Here's the drawing with two shaded views (mm, measured from the low corner). I have some questions. A direction names the side the tool comes from. Coordinates: 2 decimals unless noted, no trailing zeros. Order: outer loops, then holes, each group sorted by start corner. A loop starts at its lowest first (then second) coordinate and runs counter-clockwise, first axis right, second up. Notation, with made-up numbers: M -1.5,2 L 44.5,2 A27 cw 44.5,35 Z; hole C 21,-15.75 d11. An arc over 180 degrees is marked long. Put each result on its own line as item: value. Start each with the question number.
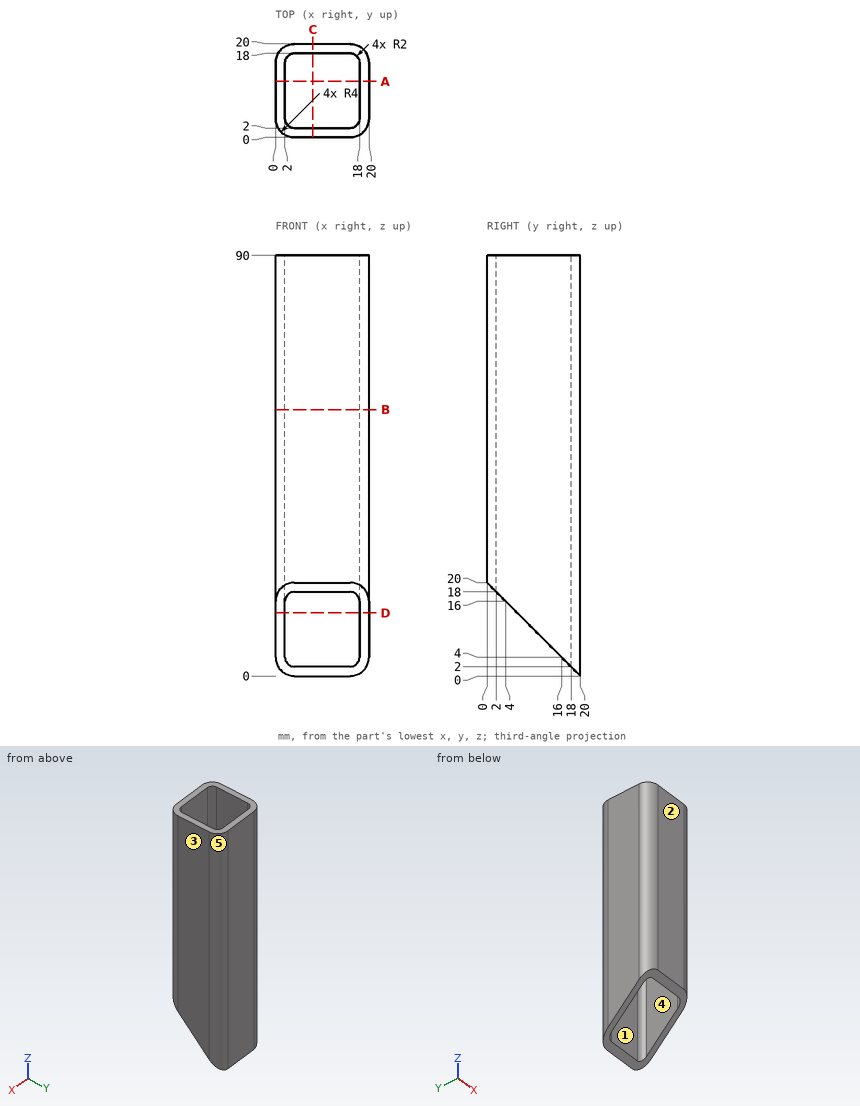
Item 1: If we section it at A-A on y = 12: Write out the boundary of the cut face in (x, z), then the cut area to 3 significant figures.
Item 2: If we section it at D-D on z = 13.5: Write out the boundary of the cut face in (x, y), then the cut area to 3 significant figures.
Item 3: If we mould it in two halves opening along Y, with no side actions, what happens to the marked faces 3, 4 and 5? For each: released by +Y, released by -Y, zero draft, split by the parting line, or undercut.
Item 4: If we section it at B-B on z = 57: Write out the boundary of the cut face in (x, y), then the cut area to 3 significant figures.
Item 5: I need wall thicknesses on probe 1 along Y at (x, z) = (4.5, 69); probe 2 along X at (y, z) = (17.75, 64.5). Which ranges of each line are inside material? Lowest first, please.
Item 6: For the marked faces 1 and 2, which set-ups out of +Z, -Z, +X, -X, +Y, -Y let a thin tool reach every point of the face, with its end or its side?
Item 7: For pin 1 Ø1.5 at (x, y) = (3.5, 13.5) entering from +Z, with a flat end and sliding along its axis, tell me the tip position at first contact or that it passes through.
Item 8: If we section it at C-C on x = 8: Write out the boundary of the cut face in (y, z).
Geometry check:
1. outline: M 0,8 L 2,8 L 2,90 L 0,90 Z; M 18,8 L 20,8 L 20,90 L 18,90 Z
1. area: 328 mm²
2. outline: M 0,6.5 L 2,6.5 L 2,16 A2 cw 4,18 L 16,18 A2 cw 18,16 L 18,6.5 L 20,6.5 L 20,16 A4 ccw 16,20 L 4,20 A4 ccw 0,16 Z
2. area: 80.8 mm²
3. face 3: zero draft
3. face 4: undercut
3. face 5: released by +Y
4. outline: M 0,4 A4 ccw 4,0 L 16,0 A4 ccw 20,4 L 20,16 A4 ccw 16,20 L 4,20 A4 ccw 0,16 Z; hole M 2,4 A2 ccw 4,2 L 16,2 A2 ccw 18,4 L 18,16 A2 ccw 16,18 L 4,18 A2 ccw 2,16 Z
4. area: 134 mm²
5. probe 1: y = 0 to 2, 18 to 20
5. probe 2: x = 0.4 to 3.03, 16.97 to 19.6
6. face 1: +Z, -Z
6. face 2: +Z, -Z, +X, -X, -Y
7. pin 1: passes through
8. outline: M 0,20 L 2,18 L 2,90 L 0,90 Z; M 18,2 L 20,0 L 20,90 L 18,90 Z
